from build123d import *

# Parameters (mm, degrees)
SKETCH1_W           = 500
SKETCH1_H           = 180
BASE_FLANGE1_DEPTH  = 3.175
FILLET1_R           = 10
SKETCH13_R          = 2.65
CUT_EXTRUDE4_DEPTH  = 266.725573901
CUT_EXTRUDE5_DEPTH  = 266.725573901
CUT_EXTRUDE6_DEPTH  = 266.725573901
SKETCH21_R          = 2.55
CUT_EXTRUDE7_DEPTH  = 10
CUT_EXTRUDE8_DEPTH  = 266.725573901
SKETCH26_R          = 3.35
CUT_EXTRUDE9_DEPTH  = 266.725573901
SKETCH27_R          = 3.35
CUT_EXTRUDE10_DEPTH = 266.725573901


# Sheet-metal steps are written as plain solids
with BuildPart() as part:
    # Sketch1 → Base-Flange1 (new body)
    with BuildSketch(Plane(origin=(0, 0, 0), x_dir=(1, 0, 0), z_dir=(0, 1, 0))):
        Rectangle(SKETCH1_W, SKETCH1_H)
    extrude(amount=-BASE_FLANGE1_DEPTH)

    # Fillet1
    fillet1_edges = [part.edges().sort_by_distance(p)[0] for p in [
        (250, -1.5875, 90),
        (-250, -1.5875, 90),
        (-250, -1.5875, -90),
        (250, -1.5875, -90),
    ]]
    fillet(fillet1_edges, radius=FILLET1_R)

    # Sketch13 → Cut-Extrude4 (cut, through all)
    with BuildSketch(Plane(origin=(0, 0, 0), x_dir=(1, 0, 0), z_dir=(0, 1, 0))):
        with Locations(Location((-135.913126074, 46.6872, 0), (0, 0, 270))):
            Circle(SKETCH13_R)
        with Locations(Location((-135.913126074, -46.6872, 0), (0, 0, 270))):
            Circle(SKETCH13_R)
        with Locations(Location((-110.913126074, -46.6872, 0), (0, 0, 270))):
            Circle(SKETCH13_R)
        with Locations(Location((-110.913126074, 46.6872, 0), (0, 0, 270))):
            Circle(SKETCH13_R)
    extrude(amount=-CUT_EXTRUDE4_DEPTH, mode=Mode.SUBTRACT)

    # Sketch15 → Cut-Extrude5 (cut, through all)
    with BuildSketch(Plane(origin=(0, 0, 0), x_dir=(1, 0, 0), z_dir=(0, 1, 0))):
        with BuildLine():
            Line((-159.413126074, -90), (-87.413126074, -90))
            Line((-87.413126074, -90), (-87.413126074, -56.5))
            ThreePointArc((-87.413126074, -56.5), (-88.877592168, -52.964466094), (-92.413126074, -51.5))
            Line((-92.413126074, -51.5), (-154.413126074, -51.5))
            ThreePointArc((-154.413126074, -51.5), (-157.94865998, -52.964466094), (-159.413126074, -56.5))
            Line((-159.413126074, -56.5), (-159.413126074, -90))
        make_face()
    cut_extrude5 = extrude(amount=-CUT_EXTRUDE5_DEPTH, mode=Mode.SUBTRACT)

    # Mirror1: Cut-Extrude5 across plane
    add(cut_extrude5.mirror(Plane.XY), mode=Mode.SUBTRACT)

    # Sketch16 → Cut-Extrude6 (cut, through all)
    with BuildSketch(Plane(origin=(0, 0, 0), x_dir=(1, 0, 0), z_dir=(0, 1, 0))):
        with BuildLine():
            Line((-82.726681877, 68.835), (-82.726681877, 73.135))
            ThreePointArc((-82.726681877, 73.135), (-80.576681877, 75.285), (-78.426681877, 73.135))
            Line((-78.426681877, 73.135), (-78.426681877, 68.835))
            ThreePointArc((-78.426681877, 68.835), (-80.576681877, 66.685), (-82.726681877, 68.835))
        make_face()
        with BuildLine():
            Line((-164.09957027, 68.835), (-164.09957027, 73.135))
            ThreePointArc((-164.09957027, 73.135), (-166.24957027, 75.285), (-168.39957027, 73.135))
            Line((-168.39957027, 73.135), (-168.39957027, 68.835))
            ThreePointArc((-168.39957027, 68.835), (-166.24957027, 66.685), (-164.09957027, 68.835))
        make_face()
    cut_extrude6 = extrude(amount=-CUT_EXTRUDE6_DEPTH, mode=Mode.SUBTRACT)

    # Sketch21 → Cut-Extrude7 (cut)
    with BuildSketch(Plane(origin=(0, 0, 0), x_dir=(1, 0, 0), z_dir=(0, 1, 0))):
        with Locations(Location((90.388844999, -24.75, 0), (0, 0, 270))):
            Circle(SKETCH21_R)
        with Locations(Location((161.611770889, -34, 0), (0, 0, 270))):
            Circle(SKETCH21_R)
        with BuildLine():
            Line((102.888844999, -27.3), (97.888844999, -27.3))
            ThreePointArc((97.888844999, -27.3), (95.338844999, -24.75), (97.888844999, -22.2))
            Line((97.888844999, -22.2), (102.888844999, -22.2))
            ThreePointArc((102.888844999, -22.2), (105.438844999, -24.75), (102.888844999, -27.3))
        make_face()
        with BuildLine():
            Line((122.145496999, -33.557591563), (102.145496999, -68.198607715))
            ThreePointArc((102.145496999, -68.198607715), (101.877690583, -69.222505113), (102.169887266, -70.239710725))
            ThreePointArc((102.169887266, -70.239710725), (161.611770889, -103.617915525), (221.053654512, -70.239710725))
            ThreePointArc((221.053654512, -70.239710725), (221.345851195, -69.222505113), (221.07804478, -68.198607715))
            Line((221.07804478, -68.198607715), (201.07804478, -33.557591563))
            ThreePointArc((201.07804478, -33.557591563), (199.863632062, -32.625739911), (198.345993972, -32.825540756))
            Line((198.345993972, -32.825540756), (170.286770889, -49.025540756))
            ThreePointArc((170.286770889, -49.025540756), (161.611770889, -51.35), (152.936770889, -49.025540756))
            Line((152.936770889, -49.025540756), (124.877547807, -32.825540756))
            ThreePointArc((124.877547807, -32.825540756), (123.359909716, -32.625739911), (122.145496999, -33.557591563))
        make_face()
    cut_extrude7 = extrude(amount=-CUT_EXTRUDE7_DEPTH, mode=Mode.SUBTRACT)

    # Mirror2: Cut-Extrude7 across plane
    add(cut_extrude7.mirror(Plane.XY), mode=Mode.SUBTRACT)

    # Mirror3: Cut-Extrude6 across plane
    add(cut_extrude6.mirror(Plane.XY), mode=Mode.SUBTRACT)

    # Sketch25 → Cut-Extrude8 (cut, through all)
    with BuildSketch(Plane(origin=(0, 0, 0), x_dir=(1, 0, 0), z_dir=(0, 1, 0))):
        with BuildLine():
            Line((127.608844999, 25), (135.608844999, 25))
            ThreePointArc((135.608844999, 25), (137.023058561, 24.414213562), (137.608844999, 23))
            Line((137.608844999, 23), (137.608844999, -23))
            ThreePointArc((137.608844999, -23), (137.023058561, -24.414213562), (135.608844999, -25))
            Line((135.608844999, -25), (127.608844999, -25))
            ThreePointArc((127.608844999, -25), (126.194631437, -24.414213562), (125.608844999, -23))
            Line((125.608844999, -23), (125.608844999, 23))
            ThreePointArc((125.608844999, 23), (126.194631437, 24.414213562), (127.608844999, 25))
        make_face()
    extrude(amount=-CUT_EXTRUDE8_DEPTH, mode=Mode.SUBTRACT)

    # Sketch26 → Cut-Extrude9 (cut, through all)
    with BuildSketch(Plane(origin=(0, 0, 0), x_dir=(1, 0, 0), z_dir=(0, 1, 0))):
        with Locations(Location((0, 0, 0), (0, 0, 270))):
            Circle(SKETCH26_R)
    extrude(amount=-CUT_EXTRUDE9_DEPTH, mode=Mode.SUBTRACT)

    # Sketch27 → Cut-Extrude10 (cut, through all)
    with BuildSketch(Plane(origin=(0, 0, 0), x_dir=(1, 0, 0), z_dir=(0, 1, 0))):
        with Locations(Location((-60, 70, 0), (0, 0, 270))):
            Circle(SKETCH27_R)
    extrude(amount=-CUT_EXTRUDE10_DEPTH, mode=Mode.SUBTRACT)


solid = part.part
The model under review builds one solid part; all positions refer to its coordinate system, in mm. A direction names the side the tool comes from. Round coordinates to 2 decimals unless told otherwise and drop trailing zeros. One line per question, with ' | ' between items. Start each with the question number.
Item 1: For pin 1 (6 mm diameter, centred on x = 90.39, z = 24.75, fed in from +Y); pin 2 (1.6 mm diameter, centred on x = 133, y = -2, fed in from -Z); pin 3 (1 mm diameter, centred on x = -128.5, y = -1, fed in from +Z), all flat-tipped, find the tip position at first contact; note any pin that passes through.
Item 2: Wall thickness on line 1 along X through (y, z) = (-1.4, 0); line 2 along X through (y, z) = (-1.2, -8); line 3 along X through (y, z) = (-2.9, 26.5): over which ranges is each line inside the solid? List them lowest first. Write a range as [from, to].
Item 3: Machinability: for faces 1 (the face through (184.513, -1.565, 40.812)), 2 (the face through (112.285, -1.565, 50.636)), 3 (the face through (184.513, -1.565, -40.812)), which of the approach directions +Z, -Z, +X, -X, +Y, -Y give a long, thin tool a straight path to every point of the face, cutting with its end or side? Answer none if there is none.
Item 4: Draft analysis for pull direction X (two halves, no side actions). For faces 4 (the face through (246.99, -1.61, 87.15)), 5 (the face through (-3.5, -3.175, -1.3)), 6 (the face through (211.22, -1.57, 51.12)), state which applies: +X half, -X half, draft (parallel to the pull), parting line (faces both ways), or undercut.
Item 5: Add section A-A, the plane y = -1. Count the separate pieces of the cut face and the enclosed holes in it, then the cut area to 3 significant figures.
Return value:
1) pin 1: stops at y = 0 | pin 2: stops at z = -37.98 | pin 3: stops at z = 51.5
2) line 1: x = [-250, -3.35], [3.35, 125.61], [137.61, 250] | line 2: x = [-250, 125.61], [137.61, 250] | line 3: x = [-250, 88.53], [92.24, 96.03], [104.74, 250]
3) face 1: +Z, +Y, -Y | face 2: +Y, -Y | face 3: -Z, +Y, -Y
4) face 4: +X half | face 5: draft | face 6: undercut
5) separate pieces: 1 | enclosed holes: 17 | area: 73,300 mm2
